Part model, mm, in its own coordinate system. Coordinates: 2 decimals unless noted, no trailing zeros. Loops run counter-clockwise (first coordinate to the right, second up) from the corner with the lowest first, then second, coordinate; pieces in that order, holes last. Notation, with made-up numbers: (-28.5, -2) - (17.5, -2) arc R16 cw to (17.5, 8) - close; hole circle Ø2 at (-27, 59.25). An arc over 180 degrees is marked (long way). Use a Markdown table: item, result. Add a question column.
1. Wall check: probe 1 along Y at (x, z) = (0, -1.1); probe 2 along X at (y, z) = (-3.25, -1.3); probe 3 along X at (y, z) = (5, -1.25). Give the ranges that are in metal, low to high. Write a range as [from, to].
2. Band-saw the part on D-D, the plane y = -2.5. Give the cut face in (x, z).
3. Band-saw the part on B-B, the plane y = 11. Give the cut face in (x, z).
4. Band-saw the part on C-C, the plane z = -0.5. Give the cut face in (x, y), plus the area to 3 significant figures.
5. Band-saw the part on A-A, the plane x = 0. Give the cut face in (y, z).
6. Pull direction X, two halves, no side cores. Call faces 1 (the flat face through (-36, 3, 0)), 2 (the cylindrical face through (-10.52, -6.26, -0.69)): pulls with the +X half, pulls with the -X half, needs draft (parallel to the pull), parting line crosses it, or undercut.
from build123d import *

# Parameters (mm, degrees)
SKETCH2_W          = 100
SKETCH2_H          = 24.5
BASE_FLANGE1_DEPTH = 1.4
SKETCH1_R          = 1.25
SKETCH1_R_2        = 6
CUT_EXTRUDE1_DEPTH = 10


# Sheet-metal steps are written as plain solids
with BuildPart() as part:
    # Sketch2 → Base-Flange1 (new body)
    with BuildSketch(Plane.XY):
        with Locations((-35, 2.75)):
            Rectangle(SKETCH2_W, SKETCH2_H)
    extrude(amount=-BASE_FLANGE1_DEPTH)

    # Sketch1 → Cut-Extrude1 (cut)
    with BuildSketch(Plane.XY):
        with Locations((0, 11)):
            Circle(SKETCH1_R)
        with Locations((-9.526279442, -5.5)):
            Circle(SKETCH1_R)
        with Locations((9.526279442, -5.5)):
            Circle(SKETCH1_R)
        Circle(SKETCH1_R_2)
    extrude(amount=-CUT_EXTRUDE1_DEPTH, mode=Mode.SUBTRACT)


solid = part.part
Geometry check:
| question | item | result |
|---|---|---|
| 1 | probe 1 | y = [-9.5, -6], [6, 9.75], [12.25, 15] |
| 1 | probe 2 | x = [-85, -5.04], [5.04, 15] |
| 1 | probe 3 | x = [-85, -3.32], [3.32, 15] |
| 2 | outline | (-85, -1.4) - (-5.45, -1.4) - (-5.45, 0) - (-85, 0) - close; (5.45, -1.4) - (15, -1.4) - (15, 0) - (5.45, 0) - close |
| 3 | outline | (-85, -1.4) - (-1.25, -1.4) - (-1.25, 0) - (-85, 0) - close; (1.25, -1.4) - (15, -1.4) - (15, 0) - (1.25, 0) - close |
| 4 | outline | (-85, -9.5) - (15, -9.5) - (15, 15) - (-85, 15) - close; hole circle Ø2.5 at (-9.53, -5.5); hole circle Ø12 at (0, 0); hole circle Ø2.5 at (0, 11); hole circle Ø2.5 at (9.53, -5.5) |
| 4 | area | 2,320 mm^2 |
| 5 | outline | (-9.5, -1.4) - (-6, -1.4) - (-6, 0) - (-9.5, 0) - close; (6, -1.4) - (9.75, -1.4) - (9.75, 0) - (6, 0) - close; (12.25, -1.4) - (15, -1.4) - (15, 0) - (12.25, 0) - close |
| 6 | face 1 | needs draft |
| 6 | face 2 | undercut |
